from build123d import *

# Parameters (mm, degrees)
SKETCH1_W                      = 127.635
SKETCH1_H                      = 127.635
MAIN_PLATE_DEPTH               = 12.7
SKETCH2_R                      = 3.556
U_BOLT_HOLE_DEPTH              = 12.7
U_BOLT_PATTERN_COUNT           = 2
U_BOLT_PATTERN_PITCH           = 34.925
U_BOLT_PATTERN_COUNT_DIR2      = 2
U_BOLT_PATTERN_PITCH_DIR2      = 89.535
SKETCH3_R                      = 1.778
RAPTOR_BOLT_HOLE_DEPTH         = 12.7
RAPTOR_BOLT_PATTERN_COUNT      = 2
RAPTOR_BOLT_PATTERN_PITCH      = 38.1
RAPTOR_BOLT_PATTERN_COUNT_DIR2 = 2
RAPTOR_BOLT_PATTERN_PITCH_DIR2 = 76.835
SKETCH4_R                      = 12.7
CO2_CYLINDER_HOLE_DEPTH        = 12.7
CO2_PATTERN_COUNT              = 2
CO2_PATTERN_PITCH              = 76.835
SKETCH5_R                      = 1.35255
FRAME_ATTACHMENT_HOLE_1_DEPTH  = 12.7
SKETCH6_R                      = 1.35255
FRAME_ATTACHMENT_HOLE_2_DEPTH  = 12.7
SKETCH7_R                      = 1.35255
FRAME_ATTACHMENT_HOLE_3_DEPTH  = 12.7
SKETCH8_R                      = 1.35255
FRAME_ATTACHMENT_HOLE_4_DEPTH  = 12.7


with BuildPart() as part:
    # Sketch1 → Main Plate (new body)
    with BuildSketch(Plane(origin=(0, 0, 0), x_dir=(1, 0, 0), z_dir=(0, 1, 0))):
        with Locations((63.8175, 63.8175)):
            Rectangle(SKETCH1_W, SKETCH1_H)
    extrude(amount=MAIN_PLATE_DEPTH)

    # Sketch2 → U-Bolt Hole (cut)
    with BuildSketch(Plane(origin=(0, 12.7, 0), x_dir=(1, 0, 0), z_dir=(0, 1, 0))):
        with Locations((46.355, 108.585)):
            Circle(SKETCH2_R)
    u_bolt_hole = extrude(amount=-U_BOLT_HOLE_DEPTH, mode=Mode.SUBTRACT)

    # U-Bolt Pattern: U-Bolt Hole 2 × 2
    with Locations(*[(i * U_BOLT_PATTERN_PITCH, 0, j * U_BOLT_PATTERN_PITCH_DIR2) for i in range(U_BOLT_PATTERN_COUNT) for j in range(U_BOLT_PATTERN_COUNT_DIR2) if (i, j) != (0, 0)]):
        add(u_bolt_hole, mode=Mode.SUBTRACT)

    # Sketch3 → Raptor Bolt Hole (cut)
    with BuildSketch(Plane(origin=(0, 12.7, 0), x_dir=(1, 0, 0), z_dir=(0, 1, 0))):
        with Locations((25.4, 44.7675)):
            Circle(SKETCH3_R)
    raptor_bolt_hole = extrude(amount=-RAPTOR_BOLT_HOLE_DEPTH, mode=Mode.SUBTRACT)

    # Raptor Bolt Pattern: Raptor Bolt Hole 2 × 2
    with Locations(*[(j * RAPTOR_BOLT_PATTERN_PITCH_DIR2, 0, -i * RAPTOR_BOLT_PATTERN_PITCH) for i in range(RAPTOR_BOLT_PATTERN_COUNT) for j in range(RAPTOR_BOLT_PATTERN_COUNT_DIR2) if (i, j) != (0, 0)]):
        add(raptor_bolt_hole, mode=Mode.SUBTRACT)

    # Sketch4 → Co2 Cylinder Hole (cut)
    with BuildSketch(Plane(origin=(0, 12.7, 0), x_dir=(1, 0, 0), z_dir=(0, 1, 0))):
        with Locations((25.4, 63.8175)):
            Circle(SKETCH4_R)
    co2_cylinder_hole = extrude(amount=-CO2_CYLINDER_HOLE_DEPTH, mode=Mode.SUBTRACT)

    # Co2 Pattern: Co2 Cylinder Hole ×2
    with Locations(*[(i * CO2_PATTERN_PITCH, 0, 0) for i in range(1, CO2_PATTERN_COUNT)]):
        add(co2_cylinder_hole, mode=Mode.SUBTRACT)

    # Sketch5 → Frame attachment hole 1 (cut)
    with BuildSketch(Plane.XY):
        with Locations((4.7625, 6.35)):
            Circle(SKETCH5_R)
    extrude(amount=-FRAME_ATTACHMENT_HOLE_1_DEPTH, mode=Mode.SUBTRACT)

    # Sketch6 → Frame attachment hole 2 (cut)
    with BuildSketch(Plane.ZY):
        with Locations((-122.8725, 6.35)):
            Circle(SKETCH6_R)
    extrude(amount=-FRAME_ATTACHMENT_HOLE_2_DEPTH, mode=Mode.SUBTRACT)

    # Sketch7 → Frame attachment hole 3 (cut)
    with BuildSketch(Plane(origin=(0, 0, -127.635), x_dir=(-1, 0, 0), z_dir=(0, 0, -1))):
        with Locations((-122.8725, 6.35)):
            Circle(SKETCH7_R)
    extrude(amount=-FRAME_ATTACHMENT_HOLE_3_DEPTH, mode=Mode.SUBTRACT)

    # Sketch8 → Frame attachment hole 4 (cut)
    with BuildSketch(Plane(origin=(127.635, 0, 0), x_dir=(0, 0, -1), z_dir=(1, 0, 0))):
        with Locations((4.7625, 6.35)):
            Circle(SKETCH8_R)
    extrude(amount=-FRAME_ATTACHMENT_HOLE_4_DEPTH, mode=Mode.SUBTRACT)


solid = part.part
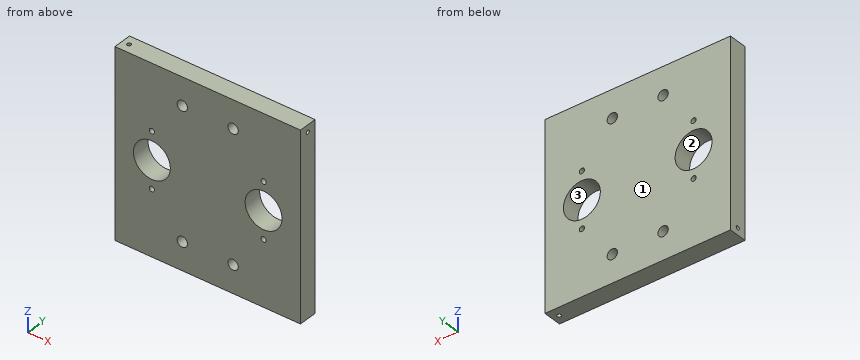
For this review, take the finished solid that the model builds, in its own axes (mm). Face numbers are marked on the shaded views. Coordinates: 2 decimals unless noted, no trailing zeros. Order: outer loops, then holes, each group sorted by start corner. A loop starts at its lowest first (then second) coordinate and runs counter-clockwise, first axis right, second up. Notation, with made-up numbers: (67.25, 89) -> (77.25, 89) arc R23 cw to (77.25, 106) -> close; hole circle Ø3 at (-36.75, 62.5). An arc over 180 degrees is marked (long way). Return JSON: item names as keys, results as strings.
1. For pin 1 Ø0.8 at (x, y) = (123.5, 6.5) entering from -Z (3 decimals); pin 2 Ø1.6 at (y, z) = (6.35, -122.87) entering from -X; pin 3 Ø15 at (x, z) = (25.4, -63.82) entering from -Y, all flat-tipped, find the tip position at first contact; note any pin that passes through.
Answer block:
{"pin 1": "z = -114.935", "pin 2": "x = 12.7", "pin 3": "through"}
2. We need section D-D on x = 96.5. Write out the cut boundary in (y, z) (3 decimals), and give its area (3 significant figures).
Answer block:
{"outline": "(0, -127.635) -> (12.7, -127.635) -> (12.7, -75.149) -> (0, -75.149) -> close; (0, -52.486) -> (12.7, -52.486) -> (12.7, 0) -> (0, 0) -> close", "area": "1,330 mm²"}
3. The part is to be moulded in two halves that separate along Z. For the marked faces 1, 2 and 3, say which applies: +Z half, -Z half, draft (parallel to the pull), parting line (faces both ways), or undercut.
Answer block:
{"face 1": "draft", "face 2": "undercut", "face 3": "undercut"}
4. We need section C-C on y = 3.5. State how many separate pieces and enclosed holes the cut face has, and give its area (3 significant figures).
Answer block:
{"separate pieces": "1", "enclosed holes": "10", "area": "15,100 mm²"}
5. We need section A-A on x = 25.4. Write out the cut boundary in (y, z) (1 decimal).
Answer block:
{"outline": "(0, -127.6) -> (12.7, -127.6) -> (12.7, -84.6) -> (0, -84.6) -> close; (0, -81.1) -> (12.7, -81.1) -> (12.7, -76.5) -> (0, -76.5) -> close; (0, -51.1) -> (12.7, -51.1) -> (12.7, -46.5) -> (0, -46.5) -> close; (0, -43) -> (12.7, -43) -> (12.7, 0) -> (0, 0) -> close"}
6. We need section B-B on z = -19.05. Write out the cut boundary in (x, y) (3 decimals), and give its area (3 significant figures).
Answer block:
{"outline": "(0, 0) -> (42.799, 0) -> (42.799, 12.7) -> (0, 12.7) -> close; (49.911, 0) -> (77.724, 0) -> (77.724, 12.7) -> (49.911, 12.7) -> close; (84.836, 0) -> (127.635, 0) -> (127.635, 12.7) -> (84.836, 12.7) -> close", "area": "1,440 mm²"}
7. For line 1 (Z direction, x = 25.4, y = 4.5) (1 decimal); line 2 (Z direction, x = 81.28, y = 3.5) (3 decimals); line 3 (X direction, y = 5.75, z = -66) (3 decimals), list the stretches that pass through material, from the lowest coordinate up. Write a range as from..to.
Answer block:
{"line 1": "-127.6..-84.6, -81.1..-76.5, -51.1..-46.5, -43..0", "line 2": "-127.635..-112.141, -105.029..-22.606, -15.494..0", "line 3": "0..12.889, 37.911..89.724, 114.746..127.635"}
